```python
from build123d import *

# Parameters (mm, degrees)
F0_R     = 31.75
F0_R_2   = 19.05
F1_DEPTH = 12.7
F2_DEPTH = 25.4
F3_D     = 19.05
F5_D     = 6.35


with BuildPart() as f1:
    # F0 (on Top) → F1 (new body)
    with BuildSketch(Plane.XY):
        Circle(F0_R)
        Circle(F0_R_2, mode=Mode.SUBTRACT)
    extrude(amount=F1_DEPTH)

    # F0 (on Top) → F2 (join)
    with BuildSketch(Plane.XY):
        Circle(F0_R_2)
    extrude(amount=F2_DEPTH)

    # F3 (through all)
    with Locations(Plane(origin=(0, 0, 0), x_dir=(1, 0, 0), z_dir=(0, 0, -1))):
        with Locations((0, 0)):
            Hole(F3_D / 2)

    # F5 (through all)
    with Locations(Plane.XY.offset(12.7)):
        with Locations((0, 25.4), (-25.4, 0), (0, -25.4), (25.4, 0)):
            Hole(F5_D / 2)


solid = f1.part
```
Could you check a few things on this model? Use its own coordinates, in mm. A direction names the side the tool comes from. Round coordinates to 2 decimals unless told otherwise and drop trailing zeros. Loops run counter-clockwise (first coordinate to the right, second up) from the corner with the lowest first, then second, coordinate; pieces in that order, holes last.
Q1. Thinking about a two-plate mould opening in X: for faces 3 (the cylindrical face through (0.41, 28.55, 6.26)), 4 (the cylindrical face through (-6.883, -30.995, 6.261)), 5 (the flat face through (7, 8, 0)), 6 (the cylindrical face through (0.41, -22.25, 6.26)), which applies, pulls with the +X half, pulls with the -X half, needs draft (parallel to the pull), parting line crosses it, or undercut?
Q2. On a 3-axis mill with a long thin cutter (end or side, diameter ignored), from which of +Z, -Z, +X, -X, +Y, -Y can I reach the whole of each face in a straight line? I mean faces 1 (the cylindrical face through (-28.43, 0.95, 6.26)), 2 (the flat face through (14, -14, 12.7)). Say none if no direction works.
Q3. I want a section at A-A (y = 0). Write out the boundary of the cut face in (x, z) (3 decimals), and give its area (3 significant figures).
Q4. For P1, Ø1, axis at x = 12, z = 4, coming from the +Y side; P2, Ø5, axis at y = -23.5, z = 9, coming from the -X side; P3, Ø8.5, axis at x = -25.4, y = 0, coming from the +Z side, each with a flat end and sliding along its axis, tell me the tip position at first contact or that it passes through.
Q5. I want a section at B-B (x = 25.4). Write out the boundary of the cut face in (y, z) (3 decimals), and give its area (3 significant figures).
Q6. Please list where these lines run through material, in increasing order: L1, parallel to Y at x = 0, z = 3.5 (3 decimals); L2, parallel to Y at x = 1.5, z = 7.5; L3, parallel to Y at x = 25.4, z = 10.25 (3 decimals).
Answer below:
1. face 3: undercut
1. face 4: parting line crosses it
1. face 5: needs draft
1. face 6: undercut
2. face 1: +Z, -Z
2. face 2: +Z
3. outline: (-31.75, 0) - (-28.575, 0) - (-28.575, 12.7) - (-31.75, 12.7) - close; (-22.225, 0) - (-9.525, 0) - (-9.525, 25.4) - (-19.05, 25.4) - (-19.05, 12.7) - (-22.225, 12.7) - close; (9.525, 0) - (22.225, 0) - (22.225, 12.7) - (19.05, 12.7) - (19.05, 25.4) - (9.525, 25.4) - close; (28.575, 0) - (31.75, 0) - (31.75, 12.7) - (28.575, 12.7) - close
3. area: 645 mm2
4. P1: stops at y = 29.59
4. P2: stops at x = -23.81
4. P3: stops at z = 12.7
5. outline: (-19.05, 0) - (-3.175, 0) - (-3.175, 12.7) - (-19.05, 12.7) - close; (3.175, 0) - (19.05, 0) - (19.05, 12.7) - (3.175, 12.7) - close
5. area: 403 mm2
6. L1: y = -31.75 to -28.575, -22.225 to -9.525, 9.525 to 22.225, 28.575 to 31.75
6. L2: y = -31.71 to -28.2, -22.6 to -9.41, 9.41 to 22.6, 28.2 to 31.71
6. L3: y = -19.05 to -3.175, 3.175 to 19.05
